Read the model definition and answer for the solid it produces. Units are mm, in the model's axes. A direction names the side the tool comes from. Round coordinates to 2 decimals unless told otherwise and drop trailing zeros. Order: outer loops, then holes, each group sorted by start corner. A loop starts at its lowest first (then second) coordinate and runs counter-clockwise, first axis right, second up. Notation, with made-up numbers: (59, -19.75) -> (114, -19.75) arc R32 cw to (114, 7.25) -> close; hole circle Ø9 at (67.5, -7). An arc over 180 degrees is marked (long way). Answer as a JSON object with one key per item and string values. Group by question number.
Item 1: Section C-C, the plane z = 137 is taken. Write down the section's boundary in (x, y).
Item 2: Section A-A, the plane x = 24.5 is taken. Write down the section's boundary in (y, z), plus the area to 3 significant figures.
Item 3: For faces 1 (the flat face through (3.2, 0.1, 200)), 2 (the flat face through (-42.675, 25.066, 1.972)), determine the directions among +Z, -Z, +X, -X, +Y, -Y from which every point of the face is accessible in a straight line to the end or side of a thin tool.
Item 4: Consider probe 1 along Z at (x, y) = (-16, -43); probe 2 along Z at (x, y) = (48, -11); probe 3 along X at (y, z) = (-4, 10.5). Determine where each line is inside the solid, lowest interval first. Write a range as from..to.
Item 5: Section B-B, the plane y = 10.5 is taken. Write down the section's boundary in (x, z), plus the area to 3 significant figures.
Item 6: The mould has two halves that part along Y. Classify faces 3 (the flat face through (0, 0, 198)), 4 (the cylindrical face through (-3, 0, 201)), 5 (the flat face through (-1, -11, 0)), 6 (the cylindrical face through (-6, 0, 98)): pulls with the +Y half, pulls with the -Y half, needs draft (parallel to the pull), parting line crosses it, or undercut.
Item 7: Given P1, Ø5, axis at x = -19.5, y = -2, coming from the +Z side; P2, Ø6, axis at x = -1.5, y = 0, coming from the -Z side, each flat-ended and moving along its own axis, determine where each tip first touches the part or whether it passes through.
from build123d import *

# Parameters (mm, degrees)
F0_R     = 7.5
F0_R_2   = 6
F1_DEPTH = 200
F2_DEPTH = 198
F0_R_3   = 47.095
F0_R_4   = 17.5
F3_DEPTH = 2
F4_DEPTH = 4
F6_R     = 3
F7_DEPTH = 2


with BuildPart() as f1:
    # F0 (on Top) → F1 (new body)
    with BuildSketch(Plane.XY):
        Circle(F0_R)
        Circle(F0_R_2, mode=Mode.SUBTRACT)
        Circle(F0_R_2)
    extrude(amount=F1_DEPTH)

    # F0 (on Top) → F2 (cut)
    with BuildSketch(Plane.XY):
        Circle(F0_R_2)
    extrude(amount=F2_DEPTH, mode=Mode.SUBTRACT)

    # F0 (on Top) → F3 (join)
    with BuildSketch(Plane.XY):
        Polygon((-32.5393686004, 42.5539186241), (-53.098972618, 7.0813562323), (-42.5539186241, -32.5393686004), (-7.0813562323, -53.098972618), (32.5393686004, -42.5539186241), (53.098972618, -7.0813562323), (42.5539186241, 32.5393686004), (7.0813562323, 53.098972618), align=None)
        Circle(F0_R_3, mode=Mode.SUBTRACT)
        Circle(F0_R_3)
        with Locations((-21.8453019556, -16.7042743772)):
            Circle(F0_R_4, mode=Mode.SUBTRACT)
        with Locations((16.7042743772, -21.8453019556)):
            Circle(F0_R_4, mode=Mode.SUBTRACT)
        with Locations((-16.7042743772, 21.8453019556)):
            Circle(F0_R_4, mode=Mode.SUBTRACT)
        Circle(F0_R, mode=Mode.SUBTRACT)
        with Locations((21.8453019556, 16.7042743772)):
            Circle(F0_R_4, mode=Mode.SUBTRACT)
    extrude(amount=F3_DEPTH)

    # F0 (on Top) → F4 (join)
    with BuildSketch(Plane.XY):
        Polygon((-32.5393686004, 42.5539186241), (-53.098972618, 7.0813562323), (-42.5539186241, -32.5393686004), (-7.0813562323, -53.098972618), (32.5393686004, -42.5539186241), (53.098972618, -7.0813562323), (42.5539186241, 32.5393686004), (7.0813562323, 53.098972618), align=None)
        Circle(F0_R_3, mode=Mode.SUBTRACT)
    extrude(amount=F4_DEPTH)

    # F6 (on offset) → F7 (join)
    with BuildSketch(Plane.XY.offset(200)):
        Circle(F6_R)
    extrude(amount=F7_DEPTH)


solid = f1.part
Values found:
{
 "1": {"outline": "circle Ø15 at (0, 0); hole circle Ø12 at (0, 0)"},
 "2": {"outline": "(-44.69, 0) -> (-37.51, 0) -> (-37.51, 2) -> (-40.22, 2) -> (-40.22, 4) -> (-44.69, 4) -> close; (-6.18, 0) -> (-0.59, 0) -> (-0.59, 2) -> (-6.18, 2) -> close; (34, 0) -> (43, 0) -> (43, 4) -> (40.22, 4) -> (40.22, 2) -> (34, 2) -> close", "area": "58.0 mm2"},
 "3": {"face 1": "+Z", "face 2": "+Z, -Z, -X, +Y"},
 "4": {"probe 1": "0..2", "probe 2": "0..4", "probe 3": "-6.34..-4.47, 4.47..6.34"},
 "5": {"outline": "(-51.12, 0) -> (-30.03, 0) -> (-30.03, 2) -> (-45.91, 2) -> (-45.91, 4) -> (-51.12, 4) -> close; (-3.38, 0) -> (5.48, 0) -> (5.48, 2) -> (-3.38, 2) -> close; (38.21, 0) -> (48.42, 0) -> (48.42, 4) -> (45.91, 4) -> (45.91, 2) -> (38.21, 2) -> close", "area": "95.8 mm2"},
 "6": {"face 3": "undercut", "face 4": "parting line crosses it", "face 5": "needs draft", "face 6": "undercut"},
 "7": {"P1": "through", "P2": "z = 198"}
}
